```python
from build123d import *

# Parameters (mm, degrees)
BOSS_EXTRUDE1_DEPTH  = 25
SKETCH3_W            = 26
SKETCH3_H            = 49
CUT_EXTRUDE1_DEPTH   = 17.2
SKETCH4_W            = 62
SKETCH4_H            = 46
CUT_EXTRUDE2_DEPTH   = 22
SKETCH5_W            = 2
SKETCH5_H            = 20
CUT_EXTRUDE4_DEPTH   = 3
SKETCH6_W            = 23
SKETCH6_H            = 15
CUT_EXTRUDE5_DEPTH   = 2
SKETCH7_W            = 35
SKETCH7_H            = 15
CUT_EXTRUDE6_DEPTH   = 6
BOSS_EXTRUDE2_DEPTH  = 1.5
SKETCH9_W            = 10
SKETCH9_H            = 0.75
CUT_EXTRUDE7_DEPTH   = 7.5
SKETCH10_W           = 1
SKETCH10_H           = 2
BOSS_EXTRUDE3_DEPTH  = 1.5
SKETCH11_W           = 1
SKETCH11_H           = 2
BOSS_EXTRUDE4_DEPTH  = 1.5
SKETCH12_W           = 2
SKETCH12_H           = 0.5
BOSS_EXTRUDE5_DEPTH  = 1
SKETCH13_W           = 2
SKETCH13_H           = 0.5
BOSS_EXTRUDE6_DEPTH  = 1
SKETCH14_W           = 2
SKETCH14_H           = 0.5
BOSS_EXTRUDE7_DEPTH  = 1
SKETCH15_W           = 2
SKETCH15_H           = 0.5
BOSS_EXTRUDE8_DEPTH  = 1
SKETCH17_W           = 2
SKETCH17_H           = 26.5
BOSS_EXTRUDE10_DEPTH = 10
SKETCH18_W           = 2
SKETCH18_H           = 26.5
BOSS_EXTRUDE11_DEPTH = 10
SKETCH19_W           = 5
SKETCH19_H           = 26.5
SKETCH19_W_2         = 4.66783526
BOSS_EXTRUDE13_DEPTH = 17.5
SKETCH20_R           = 2.5
BOSS_EXTRUDE14_DEPTH = 7
SKETCH21_R           = 1.5
CUT_EXTRUDE8_DEPTH   = 5


with BuildPart() as part:
    # Sketch2 → Boss-Extrude1 (new body)
    with BuildSketch(Plane(origin=(0, 0, 0), x_dir=(1, 0, 0), z_dir=(0, 1, 0))):
        with BuildLine():
            Line((47, -25), (-47, -25))
            ThreePointArc((-47, -25), (-49.121320344, -24.121320344), (-50, -22))
            Line((-50, -22), (-50, 22))
            ThreePointArc((-50, 22), (-49.121320344, 24.121320344), (-47, 25))
            Line((-47, 25), (47, 25))
            ThreePointArc((47, 25), (49.121320344, 24.121320344), (50, 22))
            Line((50, 22), (50, -22))
            ThreePointArc((50, -22), (49.121320344, -24.121320344), (47, -25))
        make_face()
    extrude(amount=BOSS_EXTRUDE1_DEPTH)

    # Sketch3 → Cut-Extrude1 (cut)
    with BuildSketch(Plane(origin=(0, 25, 0), x_dir=(1, 0, 0), z_dir=(0, 1, 0))):
        with Locations((34, 0)):
            Rectangle(SKETCH3_W, SKETCH3_H)
    extrude(amount=-CUT_EXTRUDE1_DEPTH, mode=Mode.SUBTRACT)

    # Sketch4 → Cut-Extrude2 (cut)
    with BuildSketch(Plane.XZ):
        with Locations((-16, 0)):
            Rectangle(SKETCH4_W, SKETCH4_H)
    extrude(amount=-CUT_EXTRUDE2_DEPTH, mode=Mode.SUBTRACT)

    # Sketch5 → Cut-Extrude4 (cut)
    with BuildSketch(Plane.ZY.offset(50)):
        with Locations((-8.75, 12.5)):
            Rectangle(SKETCH5_W, SKETCH5_H)
        with Locations((-5.25, 12.5)):
            Rectangle(SKETCH5_W, SKETCH5_H)
        with Locations((-1.75, 12.5)):
            Rectangle(SKETCH5_W, SKETCH5_H)
        with Locations((1.75, 12.5)):
            Rectangle(SKETCH5_W, SKETCH5_H)
        with Locations((5.25, 12.5)):
            Rectangle(SKETCH5_W, SKETCH5_H)
        with Locations((8.75, 12.5)):
            Rectangle(SKETCH5_W, SKETCH5_H)
    extrude(amount=-CUT_EXTRUDE4_DEPTH, mode=Mode.SUBTRACT)

    # Sketch6 → Cut-Extrude5 (cut)
    with BuildSketch(Plane(origin=(0, 0, -25), x_dir=(-1, 0, 0), z_dir=(0, 0, -1))):
        with Locations((33.5, 15.101074808)):
            Rectangle(SKETCH6_W, SKETCH6_H)
    extrude(amount=-CUT_EXTRUDE5_DEPTH, mode=Mode.SUBTRACT)

    # Sketch7 → Cut-Extrude6 (cut)
    with BuildSketch(Plane.ZY.offset(-15)):
        with Locations((0, 11.669015381)):
            Rectangle(SKETCH7_W, SKETCH7_H)
    extrude(amount=-CUT_EXTRUDE6_DEPTH, mode=Mode.SUBTRACT)

    # Sketch8 → Boss-Extrude2 (add)
    with BuildSketch(Plane(origin=(0, 25, 0), x_dir=(1, 0, 0), z_dir=(0, 1, 0))):
        with BuildLine():
            Line((-47, 25), (21, 25))
            Line((21, 25), (21, -25))
            Line((21, -25), (-47, -25))
            ThreePointArc((-47, -25), (-49.121320344, -24.121320344), (-50, -22))
            Line((-50, -22), (-50, 22))
            ThreePointArc((-50, 22), (-49.121320344, 24.121320344), (-47, 25))
        make_face()
    extrude(amount=BOSS_EXTRUDE2_DEPTH)

    # Sketch9 → Cut-Extrude7 (cut)
    with BuildSketch(Plane(origin=(21, 0, 0), x_dir=(0, 0, -1), z_dir=(1, 0, 0))):
        with Locations((0, 25.375)):
            Rectangle(SKETCH9_W, SKETCH9_H)
    extrude(amount=-CUT_EXTRUDE7_DEPTH, mode=Mode.SUBTRACT)

    # Sketch10 → Boss-Extrude3 (add)
    with BuildSketch(Plane.XZ):
        with Locations((-26.5, 24)):
            Rectangle(SKETCH10_W, SKETCH10_H)
    extrude(amount=BOSS_EXTRUDE3_DEPTH)

    # Sketch11 → Boss-Extrude4 (add)
    with BuildSketch(Plane.XZ):
        with Locations((-26.5, -24)):
            Rectangle(SKETCH11_W, SKETCH11_H)
        with Locations((26.5, 24)):
            Rectangle(SKETCH11_W, SKETCH11_H)
        with Locations((26.5, -24)):
            Rectangle(SKETCH11_W, SKETCH11_H)
    extrude(amount=BOSS_EXTRUDE4_DEPTH)

    # Sketch12 → Boss-Extrude5 (add)
    with BuildSketch(Plane.ZY.offset(27)):
        with Locations((24, -1.25)):
            Rectangle(SKETCH12_W, SKETCH12_H)
    extrude(amount=BOSS_EXTRUDE5_DEPTH)

    # Sketch13 → Boss-Extrude6 (add)
    with BuildSketch(Plane.ZY.offset(27)):
        with Locations((-24, -1.25)):
            Rectangle(SKETCH13_W, SKETCH13_H)
    extrude(amount=BOSS_EXTRUDE6_DEPTH)

    # Sketch14 → Boss-Extrude7 (add)
    with BuildSketch(Plane.ZY.offset(-26)):
        with Locations((-24, -1.25)):
            Rectangle(SKETCH14_W, SKETCH14_H)
    extrude(amount=BOSS_EXTRUDE7_DEPTH)

    # Sketch15 → Boss-Extrude8 (add)
    with BuildSketch(Plane.ZY.offset(-26)):
        with Locations((24, -1.25)):
            Rectangle(SKETCH15_W, SKETCH15_H)
    extrude(amount=BOSS_EXTRUDE8_DEPTH)

    # Sketch17 → Boss-Extrude10 (add)
    with BuildSketch(Plane.XY.offset(25)):
        with Locations((4, 13.25)):
            Rectangle(SKETCH17_W, SKETCH17_H)
    extrude(amount=BOSS_EXTRUDE10_DEPTH)

    # Sketch18 → Boss-Extrude11 (add)
    with BuildSketch(Plane(origin=(0, 0, -25), x_dir=(-1, 0, 0), z_dir=(0, 0, -1))):
        with Locations((-4, 13.25)):
            Rectangle(SKETCH18_W, SKETCH18_H)
    extrude(amount=BOSS_EXTRUDE11_DEPTH)

    # Sketch19 → Boss-Extrude13 (add)
    with BuildSketch(Plane(origin=(5, 0, 0), x_dir=(0, 0, -1), z_dir=(1, 0, 0))):
        with Locations((-32.5, 13.25)):
            Rectangle(SKETCH19_W, SKETCH19_H)
        with Locations((32.66608237, 13.25)):
            Rectangle(SKETCH19_W_2, SKETCH19_H)
    extrude(amount=BOSS_EXTRUDE13_DEPTH)

    # Sketch20 → Boss-Extrude14 (add)
    with BuildSketch(Plane.XZ.offset(-22)):
        with Locations((-40.5, 11.075)):
            Circle(SKETCH20_R)
        with Locations((8.5, 11.075)):
            Circle(SKETCH20_R)
        with Locations((-40.5, -11.075)):
            Circle(SKETCH20_R)
        with Locations((8.5, -11.075)):
            Circle(SKETCH20_R)
    extrude(amount=BOSS_EXTRUDE14_DEPTH)

    # Sketch21 → Cut-Extrude8 (cut)
    with BuildSketch(Plane(origin=(0, 15, 0), x_dir=(-1, 0, 0), z_dir=(0, -1, 0))):
        with Locations((-8.5, 11.075)):
            Circle(SKETCH21_R)
        with Locations((-8.5, -11.075)):
            Circle(SKETCH21_R)
        with Locations((40.5, 11.075)):
            Circle(SKETCH21_R)
        with Locations((40.5, -11.075)):
            Circle(SKETCH21_R)
    extrude(amount=-CUT_EXTRUDE8_DEPTH, mode=Mode.SUBTRACT)


solid = part.part
```
Verification items for the finished model (mm, model axes). A direction names the side the tool comes from. Give positions to 0.01 mm unless a question says otherwise; leave off trailing zeros. Loops run counter-clockwise (first coordinate to the right, second up) from the corner with the lowest first, then second, coordinate; pieces in that order, holes last. Notation, with made-up numbers: M -39,53 L -28,53 A26 cw -28,77 Z; hole C 70,-21 d8. An arc over 180 degrees is marked long. Return JSON: item names as keys, results as strings.
1) Section check C-C, the plane x = 8.5. Count the separate pieces of the cut face and the enclosed holes in it, and give its area (3 significant figures).
Findings:
{"separate pieces": "3", "enclosed holes": "0", "area": "609 mm2"}
2) Tool access check on faces 1 (the flat face through (5, 13, -28)), 2 (the flat face through (17, 25.75, 0)), 3 (the flat face through (-49, 12, 9.75)), 4 (the flat face through (21, 21, 0)). Record the directions out of +Z, -Z, +X, -X, +Y, -Y that give a thin tool (end or side, any length) a straight path to the whole face; none if there is none.
Findings:
{"face 1": "+X, +Y, -Y", "face 2": "+X", "face 3": "-X", "face 4": "+Y"}
3) Section check A-A, the plane x = -40.5. Enter the section's corners in (y, z) (3 decimals).
Findings:
{"outline": "M 0,-25 L 7.601,-25 L 7.601,-23 L 0,-23 Z; M 0,23 L 22,23 L 22,13.575 L 15,13.575 L 15,12.575 L 20,12.575 L 20,9.575 L 15,9.575 L 15,8.575 L 22,8.575 L 22,-8.575 L 15,-8.575 L 15,-9.575 L 20,-9.575 L 20,-12.575 L 15,-12.575 L 15,-13.575 L 22,-13.575 L 22,-23 L 22.601,-23 L 22.601,-25 L 26.5,-25 L 26.5,25 L 0,25 Z"}
4) Mould release check, pull along Z, two halves, no side actions. Record for faces 5 (the cylindrical face through (9.69, 17.46, -10.16)), 6 (the flat face through (13, 13, 35)): released by +Z, released by -Z, zero draft, split by the parting line, or undercut.
Findings:
{"face 5": "undercut", "face 6": "released by +Z"}
5) Gauge pin test, flat ends, axial feed: P1, Ø1, axis at y = 12.5, z = -23.5, coming from the -X side; P2, Ø1.5, axis at x = 36, y = 10.5, coming from the -Z side; P3, Ø2, axis at x = -4, y = 18.5, coming from the +Z side. Record the tip position at first contact, or that the pin passes through.
Findings:
{"P1": "stops at x = -49.83", "P2": "stops at z = -25", "P3": "stops at z = 25"}
6) Material ranges on L1, parallel to Z at x = -40.5, y = 18.7 (3 decimals); L2, parallel to X at y = 22.5, z = -11; L3, parallel to Z at x = 5.5, y = 17.75, recorded low to high. Write a range as [from, to].
Findings:
{"L1": "z = [-13.575, -12.575], [-9.575, -8.575], [8.575, 9.575], [12.575, 13.575], [23, 25]", "L2": "x = [-50, 21], [47, 50]", "L3": "z = [-35, -30.33], [-25, -23], [23, 25], [30, 35]"}
7) Section check B-B, the plane z = 16. Enter the section's corners in (x, y), and give its area (3 significant figures).
Findings:
{"outline": "M -50,0 L -47,0 L -47,22 L 15,22 L 15,19.17 L 21,19.17 L 21,26.5 L -50,26.5 Z; M 15,0 L 50,0 L 50,25 L 47,25 L 47,7.8 L 21,7.8 L 21,4.17 L 15,4.17 Z", "area": "705 mm2"}
